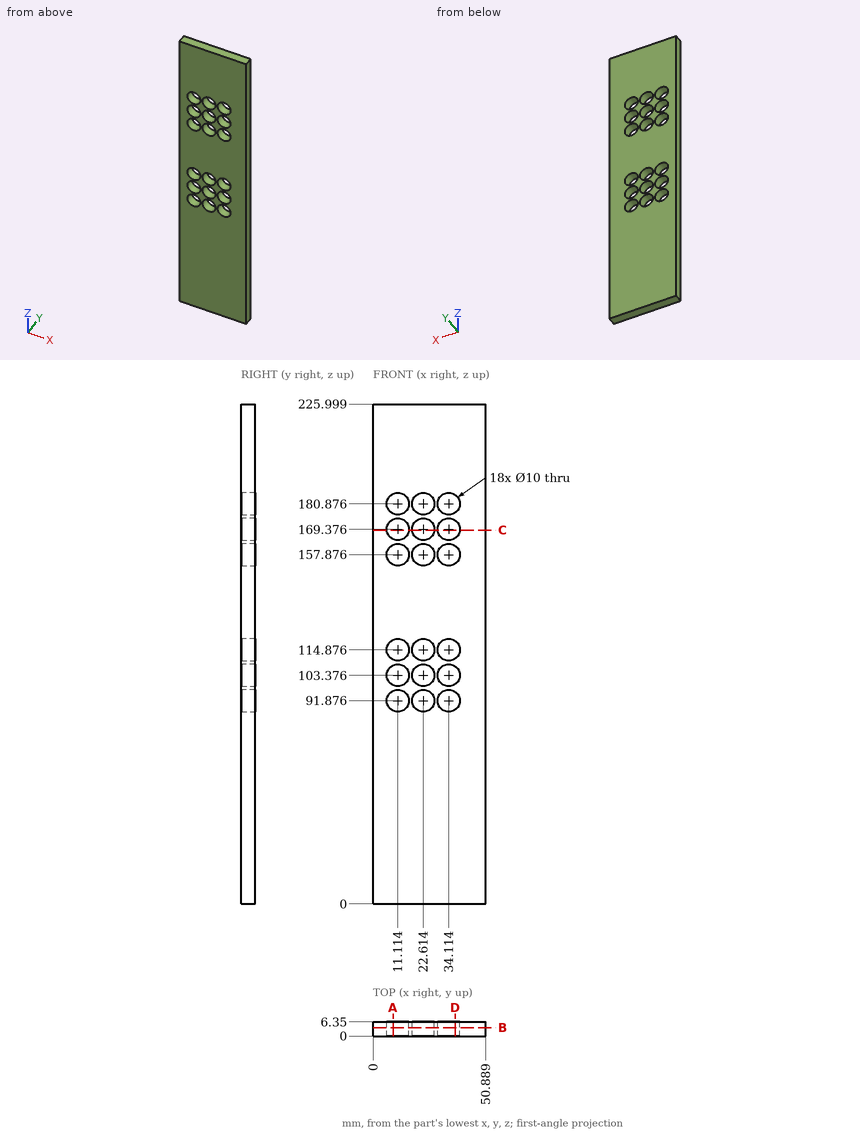
Input: dimensioned drawing with shaded views. Units: mm. Origin: part minimum x, y, z. Coordinates: 2 decimals unless noted, no trailing zeros. Write each loop counter-clockwise with the first axis right and the second up, starting at its lowest first coordinate (ties: lowest second). Pieces come first, ordered by that corner, then holes. Notation, with made-up numbers: (21, 53.5) -> (73, 53.5) arc R36 ccw to (73, 88.5) -> close; hole circle Ø1 at (-0.5, 56). An arc over 180 degrees is marked (long way). Return JSON: item names as keys, results as strings. Group by question number.
1) Section query A-A, the plane x = 9. Return loops of the section in (y, z), plus the area to 3 significant figures.
2) Ray query, line 1 along X through (y, z) = (5.25, 172); line 2 along X through (y, z) = (5, 171) (1 decimal). Return the intervals inside material, ascending.
3) Section query B-B, the plane y = 3.75. State how many separate pieces and enclosed holes the cut face has, plus the area to 3 significant figures.
4) Section query C-C, the plane z = 169. Return loops of the section in (x, y), plus the area to 3 significant figures.
5) Section query D-D, the plane x = 37. Return loops of the section in (y, z).
6) Contact query for a flat-ended pin moving along its axis: P1, Ø11.5, axis at x = 22.61, z = 103.38, coming from the +Y side. Output: stop coordinate, or through.
From the geometry:
{
 "1": {"outline": "(0, 0) -> (6.35, 0) -> (6.35, 87.34) -> (0, 87.34) -> close; (0, 96.41) -> (6.35, 96.41) -> (6.35, 98.84) -> (0, 98.84) -> close; (0, 107.91) -> (6.35, 107.91) -> (6.35, 110.34) -> (0, 110.34) -> close; (0, 119.41) -> (6.35, 119.41) -> (6.35, 153.34) -> (0, 153.34) -> close; (0, 162.41) -> (6.35, 162.41) -> (6.35, 164.84) -> (0, 164.84) -> close; (0, 173.91) -> (6.35, 173.91) -> (6.35, 176.34) -> (0, 176.34) -> close; (0, 185.41) -> (6.35, 185.41) -> (6.35, 226) -> (0, 226) -> close", "area": "1,090 mm²"},
 "2": {"line 1": "0 to 6.86, 15.37 to 18.36, 26.87 to 29.86, 38.37 to 50.89", "line 2": "0 to 6.4, 15.8 to 17.9, 27.3 to 29.4, 38.8 to 50.9"},
 "3": {"separate pieces": "1", "enclosed holes": "18", "area": "10,100 mm²"},
 "4": {"outline": "(0, 0) -> (6.13, 0) -> (6.13, 6.35) -> (0, 6.35) -> close; (16.1, 0) -> (17.63, 0) -> (17.63, 6.35) -> (16.1, 6.35) -> close; (27.6, 0) -> (29.13, 0) -> (29.13, 6.35) -> (27.6, 6.35) -> close; (39.1, 0) -> (50.89, 0) -> (50.89, 6.35) -> (39.1, 6.35) -> close", "area": "133 mm²"},
 "5": {"outline": "(0, 0) -> (6.35, 0) -> (6.35, 87.79) -> (0, 87.79) -> close; (0, 95.96) -> (6.35, 95.96) -> (6.35, 99.29) -> (0, 99.29) -> close; (0, 107.46) -> (6.35, 107.46) -> (6.35, 110.79) -> (0, 110.79) -> close; (0, 118.96) -> (6.35, 118.96) -> (6.35, 153.79) -> (0, 153.79) -> close; (0, 161.96) -> (6.35, 161.96) -> (6.35, 165.29) -> (0, 165.29) -> close; (0, 173.46) -> (6.35, 173.46) -> (6.35, 176.79) -> (0, 176.79) -> close; (0, 184.96) -> (6.35, 184.96) -> (6.35, 226) -> (0, 226) -> close"},
 "6": {"P1": "y = 6.35"}
}
